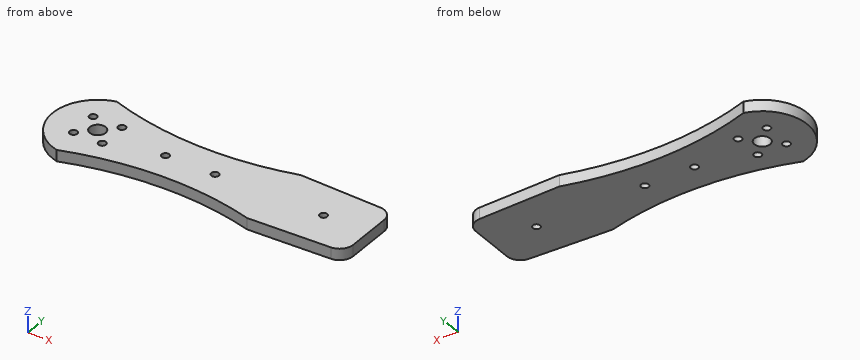
from build123d import *

# Parameters (mm, degrees)
PLASTINA_DEPTH        = 5
OTVERSTIYA_DEPTH      = 122.659652126
OTVERSTIYA_DEPTH_BACK = 122.659652126
ESKIZ_OTVERSTIYA_R    = 1.65
ESKIZ_OTVERSTIYA_R_2  = 3.5


with BuildPart() as part:
    # Eskiz_kontur → Plastina (new body)
    with BuildSketch(Plane.XY):
        with BuildLine():
            Line((78.04349, 17.26807), (114.2094, 15.99634))
            ThreePointArc((114.2094, 15.99634), (118.316039529, 14.167943464), (119.999997488, 9.999993404))
            Line((119.999997488, 9.999993404), (119.999997488, -10.000006596))
            ThreePointArc((119.999997488, -10.000006596), (118.31603808, -14.167953985), (114.2094, -15.996349022))
            Line((114.2094, -15.996349022), (78.04349, -17.268079022))
            ThreePointArc((78.04349, -17.268079022), (36.414907375, -12.045919499), (-4.891710116, -19.392564511))
            ThreePointArc((-4.891710116, -19.392564511), (-20.000005367, -4.511e-06), (-4.891710116, 19.392555489))
            ThreePointArc((-4.891710116, 19.392555489), (36.414907375, 12.045910477), (78.04349, 17.26807))
        make_face()
    extrude(amount=PLASTINA_DEPTH)

    # Eskiz_otverstiya → Otverstiya (cut, two sides: drawn at the far end of the back side and taken through both)
    with BuildSketch(Plane.XY.offset(-OTVERSTIYA_DEPTH_BACK)):
        with Locations((-6.36396, -6.36396)):
            Circle(ESKIZ_OTVERSTIYA_R)
        with Locations((6.36396, -6.36396)):
            Circle(ESKIZ_OTVERSTIYA_R)
        Circle(ESKIZ_OTVERSTIYA_R_2)
        with Locations((30, 0)):
            Circle(ESKIZ_OTVERSTIYA_R)
        with Locations((-6.36396, 6.36396)):
            Circle(ESKIZ_OTVERSTIYA_R)
        with Locations((6.36396, 6.36396)):
            Circle(ESKIZ_OTVERSTIYA_R)
        with Locations((52, 0)):
            Circle(ESKIZ_OTVERSTIYA_R)
        with Locations((100, 0)):
            Circle(ESKIZ_OTVERSTIYA_R)
    extrude(amount=OTVERSTIYA_DEPTH + OTVERSTIYA_DEPTH_BACK, mode=Mode.SUBTRACT)


solid = part.part
Verification items for the finished model (mm, model axes). Coordinates: 2 decimals unless noted, no trailing zeros. Order: outer loops, then holes, each group sorted by start corner. A loop starts at its lowest first (then second) coordinate and runs counter-clockwise, first axis right, second up.
Item 1: Section check A-A, the plane x = 52. Enter the section's corners in (y, z).
Filled in:
outline: (-12.52, 0) - (-1.65, 0) - (-1.65, 5) - (-12.52, 5) - close; (1.65, 0) - (12.52, 0) - (12.52, 5) - (1.65, 5) - close
Item 2: Depth check by flat-ended pin: pin 1 (3 mm diameter, centred on x = 26.5, z = 0.5, fed in from -Y); pin 2 (2 mm diameter, centred on x = -6.36, y = 6.36, fed in from -Z); pin 3 (1.5 mm diameter, centred on y = -12, z = 1.5, fed in from -X). Enter the tip coordinate at first touch or a pass-through.
Filled in:
pin 1: stops at y = -12.81
pin 2: passes through
pin 3: stops at x = -16.54
Item 3: Material ranges on L1, parallel to X at y = 0, z = 3.4; L2, parallel to Y at x = -7.5, z = 4.35; L3, parallel to X at y = 5, z = 1.35, recorded low to high.
Filled in:
L1: x = -20 to -3.5, 3.5 to 28.35, 31.65 to 50.35, 53.65 to 98.35, 101.65 to 120
L2: y = -18.54 to -7.56, -5.17 to 5.17, 7.56 to 18.54
L3: x = -19.36 to -7.29, -5.44 to 5.44, 7.29 to 120
Item 4: Section check C-C, the plane z = 2.7. Give the number of separate pieces and of enclosed holes in the cut face, then the cut area to 3 significant figures.
Filled in:
separate pieces: 1
enclosed holes: 8
area: 4,050 mm2
Item 5: Section check D-D, the plane x = 100. Enter the section's corners in (y, z).
Filled in:
outline: (-16.5, 0) - (-1.65, 0) - (-1.65, 5) - (-16.5, 5) - close; (1.65, 0) - (16.5, 0) - (16.5, 5) - (1.65, 5) - close
Item 6: Section check B-B, the plane y = 0. Enter the section's corners in (x, z).
Filled in:
outline: (-20, 0) - (-3.5, 0) - (-3.5, 5) - (-20, 5) - close; (3.5, 0) - (28.35, 0) - (28.35, 5) - (3.5, 5) - close; (31.65, 0) - (50.35, 0) - (50.35, 5) - (31.65, 5) - close; (53.65, 0) - (98.35, 0) - (98.35, 5) - (53.65, 5) - close; (101.65, 0) - (120, 0) - (120, 5) - (101.65, 5) - close
